Autodesk Inventor part; units mm, degrees
ref_plane "YZ Plane" through (0, 0, 0) normal (1, 0, 0) x (0, 1, 0)
ref_plane "XZ Plane" through (0, 0, 0) normal (0, 1, 0) x (-1, 0, 0)
ref_plane "XY Plane" through (0, 0, 0) normal (0, 0, 1) x (1, 0, 0)
sketch "Sketch1" plane through (0, 0, 0) normal (1, 0, 0) x (0, 1, 0)
  line L0 (3.6662, -6.35) -> (-3.6662, -6.35)
  line L1 (-3.6662, -6.35) -> (-7.3323, 0)
  line L2 (-7.3323, 0) -> (-3.6662, 6.35)
  line L3 (-3.6662, 6.35) -> (3.6662, 6.35)
  line L4 (3.6662, 6.35) -> (7.3323, 0)
  line L5 (7.3323, 0) -> (3.6662, -6.35)
  point P0 (0, 0)
  point P1 (0, 0)
  dimension "d0" = 12.7
extrude "Extrusion1" add sketch "Sketch1" along normal blind 42.5234
sketch "Sketch2" plane through (42.5234, 0, 0) normal (1, 0, 0) x (0, 0, -1)
  point P0 (0, 0)
  point P1 (0, 0)
hole "Hole1" at (42.5234, 0, 0) direction (-1, 0, 0) diameter 3.9624 depth 13.6144 tip angle 118
sketch "Sketch3" plane through (0, 0, 0) normal (-1, 0, 0) x (0, 0, 1)
  point P0 (0, 0)
  point P1 (0, 0)
hole "Hole2" at (0, 0, 0) direction (1, 0, 0) diameter 3.9624 depth 13.6144 tip angle 118
properties part number "STOCK,HEX,SHAFT,KICKER,REVERSER"
Read the model definition and answer for the solid it produces. Units are mm, in the model's axes. A direction names the side the tool comes from. Coordinates: 2 decimals unless noted, no trailing zeros. Loops run counter-clockwise (first coordinate to the right, second up) from the corner with the lowest first, then second, coordinate; pieces in that order, holes last. Notation, with made-up numbers: (-15, 26) - (1, 26) arc R26 ccw to (1, 50) - close; hole circle Ø9 at (64, 42). An arc over 180 degrees is marked (long way). Answer in a Markdown table with one row per item.
Q1. Given P1, Ø3, axis at y = 0, z = 0, coming from the -X side; P2, Ø3, axis at x = 19.5, z = 2, coming from the +Y side; P3, Ø1, axis at x = 21, z = 1.5, coming from the +Y side, each flat-ended and moving along its own axis, determine where each tip first touches the part or whether it passes through.
Here are the results:
| item | result |
|---|---|
| P1 | stops at x = 13.9 |
| P2 | stops at y = 7.04 |
| P3 | stops at y = 6.75 |
Q2. Find section A-A on x = 7. Write down the section's boundary in (y, z), plus the area to 3 significant figures.
Here are the results:
| item | result |
|---|---|
| outline | (-7.33, 0) - (-3.67, -6.35) - (3.67, -6.35) - (7.33, 0) - (3.67, 6.35) - (-3.67, 6.35) - close; hole circle Ø3.96 at (0, 0) |
| area | 127 mm^2 |
Q3. For faces 1 (the flat face through (21, 0, 6.35)), 2 (the cylindrical face through (35.621, -1.964, 0.258)), determine the directions among +Z, -Z, +X, -X, +Y, -Y from which every point of the face is accessible in a straight line to the end or side of a thin tool.
Here are the results:
| item | result |
|---|---|
| face 1 | +Z, +X, -X, +Y, -Y |
| face 2 | +X |
Q4. Find section D-D on y = 4.75. Write down the section's boundary in (x, z).
Here are the results:
| item | result |
|---|---|
| outline | (0, -4.47) - (42.52, -4.47) - (42.52, 4.47) - (0, 4.47) - close |
Q5. Straight lines are drawn through the part: line 1 along Z through (x, y) = (4.75, 0); line 2 along Y through (x, z) = (8.25, 0); line 3 along Z through (x, y) = (20, -4.5). For each, find the intervals that lie inside material, in ascending order. Write a range as [from, to].
Here are the results:
| item | result |
|---|---|
| line 1 | z = [-6.35, -1.98], [1.98, 6.35] |
| line 2 | y = [-7.33, -1.98], [1.98, 7.33] |
| line 3 | z = [-4.91, 4.91] |
Q6. Find section C-C on z = -4.25. Write down the section's boundary in (x, y), plus the area to 3 significant figures.
Here are the results:
| item | result |
|---|---|
| outline | (0, -4.88) - (42.52, -4.88) - (42.52, 4.88) - (0, 4.88) - close |
| area | 415 mm^2 |
Q7. Find section B-B on x = 18. Write down the section's boundary in (y, z).
Here are the results:
| item | result |
|---|---|
| outline | (-7.33, 0) - (-3.67, -6.35) - (3.67, -6.35) - (7.33, 0) - (3.67, 6.35) - (-3.67, 6.35) - close |
Q8. The mould has two halves that part along Y. Classify faces 3 (the flat face through (0, 2, 2)), 4 (the cylindrical face through (6.903, -1.964, -0.258)), 5 (the flat face through (20.964, 5.525, -3.131)), 6 (the conical face through (27.925, 0.103, -0.328)): pulls with the +Y half, pulls with the -Y half, needs draft (parallel to the pull), parting line crosses it, or undercut.
Here are the results:
| item | result |
|---|---|
| face 3 | needs draft |
| face 4 | undercut |
| face 5 | pulls with the +Y half |
| face 6 | undercut |
